Work out the finished part from the listing and answer in its coordinate system (mm). A direction names the side the tool comes from. Round coordinates to 2 decimals unless told otherwise and drop trailing zeros. Write each loop counter-clockwise with the first axis right and the second up, starting at its lowest first coordinate (ties: lowest second). Pieces come first, ordered by that corner, then holes.
1. Flat-ended cylindrical pins translate along their axes: pin 1 Ø1.6 at (y, z) = (91, 44.5) entering from +X; pin 2 Ø6 at (y, z) = (54, 24) entering from +X; pin 3 Ø6 at (x, y) = (13, 36) entering from +Z. Find the tip coordinate at first contact, or state that the pin passes through.
2. A tool of negligible diameter and unlimited length cuts with its end or side. For faces 1 (the face through (-39, 88.9, -22)), 2 (the face through (25.4, 25, 22)), 3 (the face through (42.936, 90.465, -15.013)), 4 (the face through (0, 14.853, 42)), from which of +Z, -Z, +X, -X, +Y, -Y can it reach the whole face along a straight path? Write none if from no direction.
3. Find section B-B (y = 62). Write down the section's boundary in (x, z), and give its area (3 significant figures).
4. Straight lines are drawn through the part: probe 1 along Z at (x, y) = (0, 97.5) (3 decimals); probe 2 along Z at (x, y) = (0, 90) (3 decimals); probe 3 along Y at (x, z) = (-2, 30). For each, find the intervals that lie inside material, in ascending order.
5. Find section A-A (x = 0). Count the separate pieces of the cut face and the enclosed holes in it, and give its area (3 significant figures).
6. Determine the mould class of faces 5 (the face through (-3.637, 56.883, -27.697)), 6 (the face through (-0.1, 0, 22.5)), 7 (the face through (-5.37, 57.52, 24.17)) for opening direction X: pulls with the +X half, pulls with the -X half, needs draft (parallel to the pull), parting line crosses it, or undercut.
```python
from build123d import *
from build123d.topology import SkipClean

# Parameters (mm, degrees)
SHELL1_T                = -3.175
BOSS_EXTRUDE1_START     = -3.175
BOSS_EXTRUDE1_DEPTH     = 3.175
CIRPATTERN1_COUNT       = 3
SKETCH4_W               = 50.8
SKETCH4_H               = 25.4
BOSS_EXTRUDE2_DEPTH     = 44.45
CUT_EXTRUDE1_DEPTH      = 87.342151299
CUT_EXTRUDE1_DEPTH_BACK = 87.342151299
SKETCH5_R               = 22.225
SKETCH6_W               = 45.72
SKETCH6_H               = 21.336
CUT_EXTRUDE2_DEPTH      = 40.767
BOSS_EXTRUDE3_DEPTH     = 1.905
SKETCH8_W               = 45.72
SKETCH8_H               = 1.905
BOSS_EXTRUDE4_DEPTH     = 16.256
SKETCH10_R              = 41.275
SKETCH10_R_2            = 38.1
BOSS_EXTRUDE5_DEPTH     = 9.525


with BuildPart() as part:
    # Sketch1 → Revolve1 (revolve)
    with BuildSketch(Plane.XY, mode=Mode.PRIVATE) as revolve1_sk:
        Polygon((0, 92.075), (-41.275, 92.075), (-41.275, 88.9), (-25.4, 50.8), (-25.4, 0), (0, 0), align=None)
    revolve(revolve1_sk.sketch.rotate(Axis((0, 0, 0), (0, 1, 0)), 180), axis=Axis((0, 0, 0), (0, 1, 0)))

    # Shell1
    shell1_openings = [part.faces().sort_by_distance(p)[0] for p in [
        (0, 0, 0),
        (0, 92.075, 0),
    ]]
    offset(amount=SHELL1_T, openings=shell1_openings, kind=Kind.INTERSECTION)

    # Sketch2 → Boss-Extrude1 (add)
    with BuildSketch(Plane(origin=(0, 92.075, 0), x_dir=(1, 0, 0), z_dir=(0, 1, 0)).offset(BOSS_EXTRUDE1_START)):
        with BuildLine():
            Line((0, -48.863958414), (-8.466666667, -48.863958414))
            Line((-8.466666667, -48.863958414), (-8.466666667, -40.397291748))
            ThreePointArc((-8.466666667, -40.397291748), (0, -41.275), (8.466666667, -40.397291748))
            Line((8.466666667, -40.397291748), (8.466666667, -48.863958414))
            Line((8.466666667, -48.863958414), (0, -48.863958414))
        make_face()
    boss_extrude1 = extrude(amount=BOSS_EXTRUDE1_DEPTH)

    # CirPattern1: Boss-Extrude1 ×3 about axis
    cirpattern1_axis = Axis((0, 0, 0), (0, 1, 0))
    for i in range(1, CIRPATTERN1_COUNT):
        add(boss_extrude1.rotate(cirpattern1_axis, i * 360 / CIRPATTERN1_COUNT))

    # Sketch4 → Boss-Extrude2 (add)
    with BuildSketch(Plane.XY):
        with Locations((0, 25.520500134)):
            Rectangle(SKETCH4_W, SKETCH4_H)
    extrude(amount=BOSS_EXTRUDE2_DEPTH)

    # Sketch5 → Cut-Extrude1 (cut, two sides: drawn at the far end of the back side and taken through both)
    with BuildSketch(Plane(origin=(0, 38.220500134, 0), x_dir=(1, 0, 0), z_dir=(0, 1, 0)).offset(-CUT_EXTRUDE1_DEPTH_BACK)):
        with Locations(Location((0, 0, 0), (0, 0, 180))):
            Circle(SKETCH5_R)
    extrude(amount=CUT_EXTRUDE1_DEPTH + CUT_EXTRUDE1_DEPTH_BACK, mode=Mode.SUBTRACT)

    # Sketch6 → Cut-Extrude2 (cut)
    with BuildSketch(Plane.XY.offset(44.45)):
        with Locations((0, 25.520500134)):
            Rectangle(SKETCH6_W, SKETCH6_H)
    extrude(amount=-CUT_EXTRUDE2_DEPTH, mode=Mode.SUBTRACT)

    # Sketch7 → Boss-Extrude3 (add)
    with SkipClean():  # the faces are left unmerged after this step: merging them gives an invalid solid
        with BuildSketch(Plane(origin=(0, 14.852500134, 0), x_dir=(1, 0, 0), z_dir=(0, 1, 0))):
            with BuildLine():
                Line((0, -22.860352775), (-22.86, -22.860352775))
                Line((-22.86, -22.860352775), (-22.860352775, 0))
                Line((-22.860352775, 0), (-22.225, 0))
                ThreePointArc((-22.225, 0), (-1.847898428, -22.148044979), (21.917712837, -3.683))
                Line((21.917712837, -3.683), (22.86, -3.683))
                Line((22.86, -3.683), (22.860352775, 0))
                Line((22.860352775, 0), (22.86, -22.860352775))
                Line((22.86, -22.860352775), (0, -22.860352775))
            make_face()
        extrude(amount=BOSS_EXTRUDE3_DEPTH)

    # Sketch8 → Boss-Extrude4 (add)
    with SkipClean():  # the faces are left unmerged after this step: merging them gives an invalid solid
        with BuildSketch(Plane.XY.offset(22.860352775)):
            with Locations((0, 15.805000134)):
                Rectangle(SKETCH8_W, SKETCH8_H)
        extrude(amount=BOSS_EXTRUDE4_DEPTH)

    # Sketch10 → Boss-Extrude5 (add)
    with BuildSketch(Plane(origin=(0, 92.075, 0), x_dir=(1, 0, 0), z_dir=(0, 1, 0))):
        with Locations(Location((0, 0, 0), (0, 0, 18.162995844))):
            Circle(SKETCH10_R)
        with Locations(Location((0, 0, 0), (0, 0, 180))):
            Circle(SKETCH10_R_2, mode=Mode.SUBTRACT)
    extrude(amount=BOSS_EXTRUDE5_DEPTH)


solid = part.part
```
Worked answers:
1. pin 1: stops at x = 8.47
1. pin 2: stops at x = 17.04
1. pin 3: stops at z = 44.45
2. face 1: -Z, -X, -Y
2. face 2: +Z, -Z, +X, -Y
2. face 3: +X, +Y, -Y
2. face 4: +Z
3. outline: circle Ø60.13 at (0, 0); hole circle Ø53.25 at (0, 0)
3. area: 613 mm2
4. probe 1: z = -41.275 to -38.1, 38.1 to 41.275
4. probe 2: z = -41.275 to -38.1, 38.1 to 48.864
4. probe 3: y = 12.82 to 16.76, 36.19 to 38.22, 62 to 70.25
5. separate pieces: 3
5. enclosed holes: 0
5. area: 731 mm2
6. face 5: parting line crosses it
6. face 6: needs draft
6. face 7: undercut
